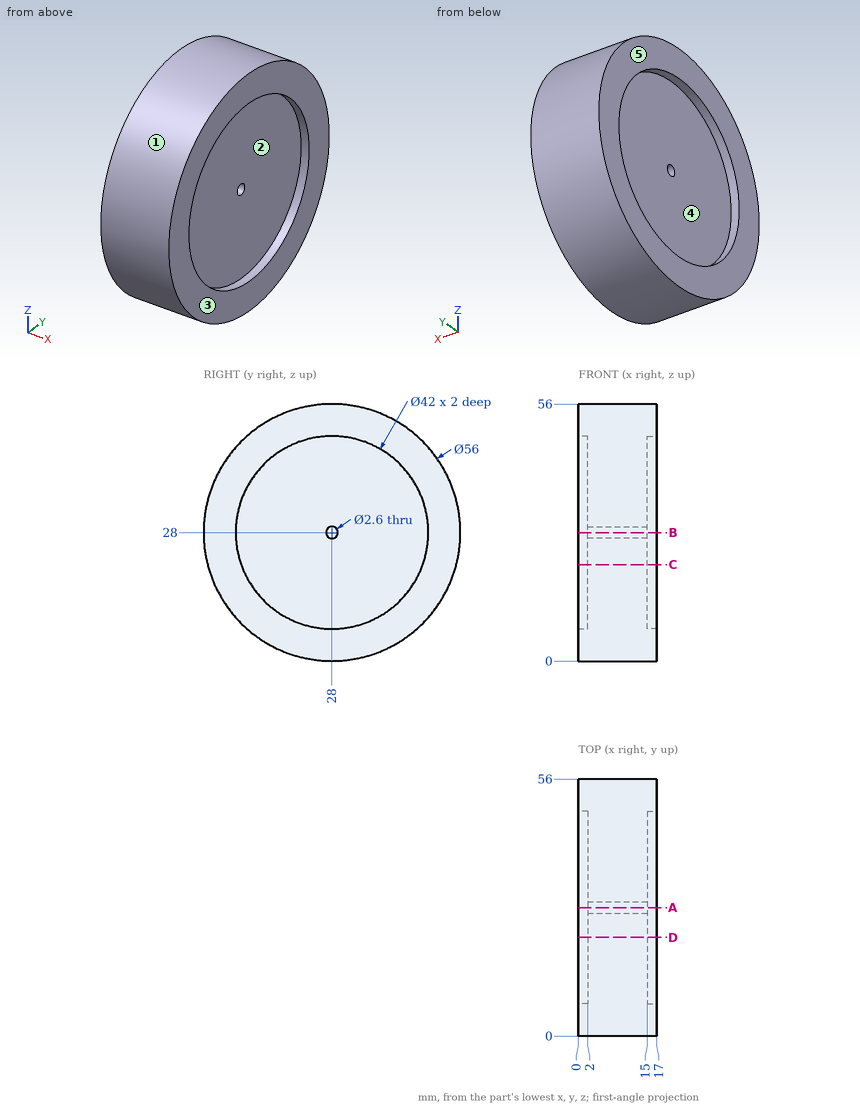
The figure shows three views and two pictorial views of one solid part (mm, origin at its lowest corner). Answer the questions. A direction names the side the tool comes from. Coordinates: 2 decimals unless noted, no trailing zeros. Loops run counter-clockwise (first coordinate to the right, second up) from the corner with the lowest first, then second, coordinate; pieces in that order, holes last. Notation, with made-up numbers: (69, 33.25) - (96, 33.25) arc R6 ccw to (96, 40.25) - close; hole circle Ø11 at (23.25, 65). An arc over 180 degrees is marked (long way). Answer in a Markdown table with one row per item.
Q1. Given P1, Ø1.5, axis at y = 28, z = 42, coming from the -X side; P2, Ø1.5, axis at x = 6, y = 38, coming from the +Z side; P3, Ø5, axis at x = 5.5, y = 34.5, coming from the -Z side, each flat-ended and moving along its own axis, determine where each tip first touches the part or whether it passes through.
Here are the results:
| item | result |
|---|---|
| P1 | stops at x = 2 |
| P2 | stops at z = 54.43 |
| P3 | stops at z = 0.29 |
Q2. For the marked faces 4 and 5, determine the directions among +Z, -Z, +X, -X, +Y, -Y from which every point of the face is accessible in a straight line to the end or side of a thin tool.
Here are the results:
| item | result |
|---|---|
| face 4 | -X |
| face 5 | +Z, -Z, -X, +Y, -Y |
Q3. Find section C-C on z = 21. Write down the section's boundary in (x, y).
Here are the results:
| item | result |
|---|---|
| outline | (0, 0.89) - (17, 0.89) - (17, 8.2) - (15, 8.2) - (15, 47.8) - (17, 47.8) - (17, 55.11) - (0, 55.11) - (0, 47.8) - (2, 47.8) - (2, 8.2) - (0, 8.2) - close |
Q4. Find section D-D on y = 21.5. Write down the section's boundary in (x, z), plus the area to 3 significant figures.
Here are the results:
| item | result |
|---|---|
| outline | (0, 0.76) - (17, 0.76) - (17, 8.03) - (15, 8.03) - (15, 47.97) - (17, 47.97) - (17, 55.24) - (0, 55.24) - (0, 47.97) - (2, 47.97) - (2, 8.03) - (0, 8.03) - close |
| area | 766 mm^2 |
Q5. Find section A-A on y = 28. Write down the section's boundary in (x, z), plus the area to 3 significant figures.
Here are the results:
| item | result |
|---|---|
| outline | (0, 0) - (17, 0) - (17, 7) - (15, 7) - (15, 26.7) - (2, 26.7) - (2, 7) - (0, 7) - close; (0, 49) - (2, 49) - (2, 29.3) - (15, 29.3) - (15, 49) - (17, 49) - (17, 56) - (0, 56) - close |
| area | 750 mm^2 |
Q6. The mould has two halves that part along Z. Classify the marked faces 1, 2 and 3: pulls with the +Z half, pulls with the -Z half, needs draft (parallel to the pull), parting line crosses it, or undercut.
Here are the results:
| item | result |
|---|---|
| face 1 | parting line crosses it |
| face 2 | undercut |
| face 3 | needs draft |
Q7. Straight lines are drawn through the part: line 1 along Y through (x, z) = (16.5, 28); line 2 along X through (y, z) = (21, 40.5); line 3 along Y through (x, z) = (13, 29). For each, find the intervals that lie inside material, in ascending order. Write a range as [from, to].
Here are the results:
| item | result |
|---|---|
| line 1 | y = [0, 7], [49, 56] |
| line 2 | x = [2, 15] |
| line 3 | y = [0.02, 27.17], [28.83, 55.98] |
